```python
from build123d import *

# Parameters (mm, degrees)
SKETCH1_W           = 19.05
SKETCH1_H           = 76.2
SKETCH1_R           = 3.81
SKETCH1_W_2         = 12.827
SKETCH1_H_2         = 3.302
BOSS_EXTRUDE1_DEPTH = 3.175
FILLET1_R           = 8.89
FILLET2_R           = 8.89


with BuildPart() as part:
    # Sketch1 → Boss-Extrude1 (new body)
    with BuildSketch(Plane(origin=(0, 0, 0), x_dir=(1, 0, 0), z_dir=(0, 1, 0))):
        Rectangle(SKETCH1_W, SKETCH1_H)
        with Locations((0, 25.4)):
            Circle(SKETCH1_R, mode=Mode.SUBTRACT)
        with Locations((0, -8.001)):
            Rectangle(SKETCH1_W_2, SKETCH1_H_2, mode=Mode.SUBTRACT)
    extrude(amount=BOSS_EXTRUDE1_DEPTH)

    # Fillet1
    fillet1_edges = [part.edges().sort_by_distance(p)[0] for p in [
        (9.525, 1.5875, -38.1),
    ]]
    fillet(fillet1_edges, radius=FILLET1_R)

    # Fillet2
    fillet2_edges = [part.edges().sort_by_distance(p)[0] for p in [
        (-9.525, 1.5875, -38.1),
    ]]
    fillet(fillet2_edges, radius=FILLET2_R)


solid = part.part
```
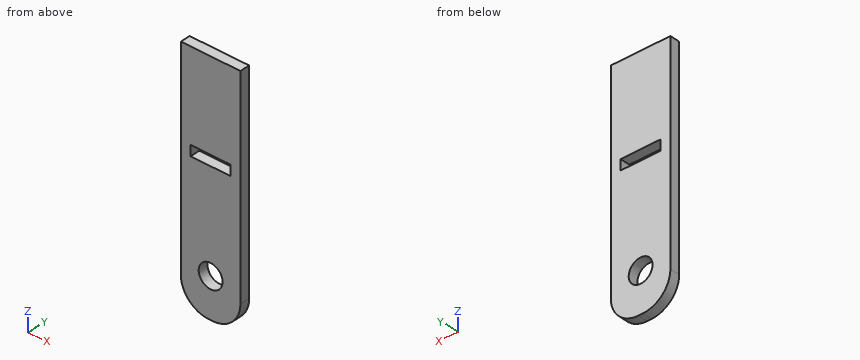
Work out the finished part from the listing and answer in its coordinate system (mm). Round coordinates to 2 decimals unless told otherwise and drop trailing zeros. Loops run counter-clockwise (first coordinate to the right, second up) from the corner with the lowest first, then second, coordinate; pieces in that order, holes last. Notation, with made-up numbers: M 66.5,-36 L 108.5,-36 A5 cw 108.5,-30 Z; hole C -11.75,0 d7. An arc over 180 degrees is marked long. One line per question, with ' | ' between items.
Q1. Find section C-C, the plane x = 0. Give the vertices of the cut face in (y, z) (3 decimals), then the cut area to 3 significant figures.
Conclusion:
outline: M 0,-38.1 L 3.175,-38.1 L 3.175,-29.21 L 0,-29.21 Z; M 0,-21.59 L 3.175,-21.59 L 3.175,6.35 L 0,6.35 Z; M 0,9.652 L 3.175,9.652 L 3.175,38.1 L 0,38.1 Z | area: 207 mm2
Q2. This flat-tipped pin is pushed along its axis until it touches: pin 1 Ø7 at (x, z) = (0, -25.4) entering from +Y. Where does it stop, or does it pass through?
Conclusion:
pin 1: passes through
Q3. Find section B-B, the plane y = 1.75. State how many separate pieces and enclosed holes the cut face has, then the cut area to 3 significant figures.
Conclusion:
separate pieces: 1 | enclosed holes: 2 | area: 1,330 mm2
Q4. Consider line 1 along Z through (x, y) = (0, 0.85); line 2 along X through (y, z) = (1.75, -25.4) (3 decimals); line 3 along Z through (x, y) = (-1.5, 1.95). Determine where each line is inside the solid, lowest interval first. Write a range as from..to.
Conclusion:
line 1: z = -38.1..-29.21, -21.59..6.35, 9.65..38.1 | line 2: x = -9.525..-3.81, 3.81..9.525 | line 3: z = -38.06..-28.9, -21.9..6.35, 9.65..38.1
Q5. Find section A-A, the plane z = -25.4. Give the vertices of the cut face in (x, y) (3 decimals).
Conclusion:
outline: M -9.525,0 L -3.81,0 L -3.81,3.175 L -9.525,3.175 Z; M 3.81,0 L 9.525,0 L 9.525,3.175 L 3.81,3.175 Z
